from build123d import *

# Parameters (mm, degrees)
F1_R          = 12.6
F2_DEPTH      = 11.25
F2_DEPTH_BACK = 11.25
F3_SIZE       = 1.5


with BuildPart() as f2:
    # F1 (on face) → F2 (new body, two sides)
    with BuildSketch(Plane.YZ) as f2_sk:
        with BuildLine():
            Line((129.016359, 24.99787), (128.36368, 24.99787))
            Line((128.36368, 24.99787), (0.32634, 24.99787))
            Line((0.32634, 24.99787), (-0.32634, 24.99787))
            ThreePointArc((-0.32634, 24.99787), (-24.999467, -0.163173), (0, -25))
            Line((0, -25), (128.690019, -25))
            ThreePointArc((128.690019, -25), (153.689487, -0.163173), (129.016359, 24.99787))
        make_face()
        Circle(F1_R, mode=Mode.SUBTRACT)
        with Locations((128.690019, 0)):
            Circle(F1_R, mode=Mode.SUBTRACT)
    extrude(amount=F2_DEPTH)
    extrude(f2_sk.sketch, amount=-F2_DEPTH_BACK)

    # F3
    f3_edges = [f2.edges().sort_by_distance(p)[0] for p in [
        (-11.25, 116.090019, 0),
        (-11.25, 153.689487, -0.163173),
        (-11.25, 64.34501, -25),
        (-11.25, 64.34501, 24.99787),
        (-11.25, -12.6, 0),
        (11.25, 64.34501, 24.99787),
        (11.25, -24.999467, -0.163173),
        (11.25, -12.6, 0),
        (0, 12.6, 0),
        (11.25, 116.090019, 0),
    ]]
    chamfer(f3_edges, length=F3_SIZE)


solid = f2.part
Work out the finished part from the listing and answer in its coordinate system (mm). Give positions to 0.01 mm unless a question says otherwise; leave off trailing zeros. Order: outer loops, then holes, each group sorted by start corner. A loop starts at its lowest first (then second) coordinate and runs counter-clockwise, first axis right, second up. Notation, with made-up numbers: (-15.75, 57.5) -> (36.25, 57.5) arc R8 ccw to (36.25, 61.5) -> close; hole circle Ø1 at (57, -16.75). An arc over 180 degrees is marked (long way). Answer as a JSON object with one key per item and string values. Group by question number.
1. Section A-A on z = 0 is taken. Determine the outline of the cut face in (x, y), plus the area to 3 significant figures.
2. Consider line 1 along Z through (x, y) = (4.5, 0); line 2 along Y through (x, z) = (-9, 6.5); line 3 along Y through (x, z) = (1, 1). Determine where each line is inside the solid, lowest interval first. Write a range as [from, to].
3. Flat-ended cylindrical pins translate along their axes: pin 1 Ø5 at (x, z) = (0.5, -18.5) entering from -Y; pin 2 Ø4 at (x, z) = (6.5, -18) entering from +Y; pin 3 Ø5 at (y, z) = (129.5, 11) entering from +X. Find the tip coordinate at first contact, or state that the pin passes through.
4. Section B-B on x = 8 is taken. Determine the outline of the cut face in (y, z), plus the area to 3 significant figures.
Result sheet:
{
 "1": {"outline": "(-11.25, -23.5) -> (-9.75, -25) -> (9.75, -25) -> (11.25, -23.5) -> (11.25, -14.1) -> (9.75, -12.6) -> (-9.75, -12.6) -> (-11.25, -14.1) -> close; (-11.25, 14.1) -> (-9.75, 12.6) -> (9.75, 12.6) -> (11.25, 14.1) -> (11.25, 114.59) -> (9.75, 116.09) -> (-9.75, 116.09) -> (-11.25, 114.59) -> close; (-11.25, 142.79) -> (-9.75, 141.29) -> (9.75, 141.29) -> (11.25, 142.79) -> (11.25, 152.19) -> (9.75, 153.69) -> (-9.75, 153.69) -> (-11.25, 152.19) -> close", "area": "2,870 mm^2"},
 "2": {"line 1": "z = [-25, -12.6], [12.6, 25]", "line 2": "y = [-24.14, -10.79], [10.79, 117.9], [139.48, 152.83]", "line 3": "y = [-24.98, -12.56], [12.56, 116.13], [141.25, 153.67]"},
 "3": {"pin 1": "stops at y = -19.21", "pin 2": "stops at y = 147.9", "pin 3": "stops at x = 10.68"},
 "4": {"outline": "(-0.33, 25) arc R25 ccw to (0, -25) -> (128.69, -25) arc R25 ccw to (129.02, 25) -> close; hole circle Ø25.2 at (0, 0); hole circle Ø25.2 at (128.69, 0)", "area": "7,400 mm^2"}
}
